For this review, take the finished solid that the model builds, in its own axes (mm). Face numbers are marked on the shaded views. A direction names the side the tool comes from. Round coordinates to 2 decimals unless told otherwise and drop trailing zeros. Loops run counter-clockwise (first coordinate to the right, second up) from the corner with the lowest first, then second, coordinate; pieces in that order, holes last. Notation, with made-up numbers: (4, -5) -> (49, -5) arc R27 cw to (49, 32) -> close; hole circle Ø1 at (-15.75, 45.5). An arc over 180 degrees is marked (long way). Write each question's results on one line, items separated by ' | '.
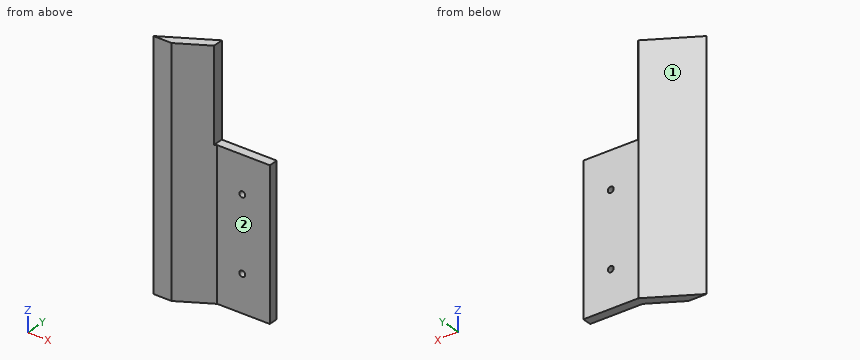
Autodesk Inventor part; units mm, degrees
ref_plane "YZ Plane" through (0, 0, 0) normal (1, 0, 0) x (0, 1, 0)
ref_plane "XZ Plane" through (0, 0, 0) normal (0, 1, 0) x (-1, 0, 0)
ref_plane "XY Plane" through (0, 0, 0) normal (0, 0, 1) x (1, 0, 0)
sketch "スケッチ1" plane through (0, 0, 0) normal (0, 0, 1) x (1, 0, 0)
  line L0 (0, 0) -> (25.9808, 15)
  line L1 (25.9808, 15) -> (55.9808, 15)
  line L2 (55.9808, 15) -> (55.9808, 10)
  line L3 (55.9808, 10) -> (27.3205, 10)
  line L4 (27.3205, 10) -> (10, 0)
  line L5 (10, 0) -> (0, 0)
  dimension "d0" = 15
  dimension "d1" = 5
  dimension "d2" = 5
  dimension "d3" = 30
  dimension "d21" = 30
extrude "押し出し1" add sketch "スケッチ1" along normal blind 130
sketch "スケッチ2" plane through (25.9808, 15, 0) normal (0, 1, 0) x (1, 0, 0)
  line L0 (0.0508, -80) -> (34.0508, -80)
  line L1 (34.0508, -80) -> (34.0508, -130.8394)
  line L2 (34.0508, -130.8394) -> (0.0508, -130.8394)
  line L3 (0.0508, -130.8394) -> (0.0508, -80)
  line L4 (30, 0) -> (0, 0)
  line L5 (30, -130) -> (0, -130)
  point P0 (-25.9808, 0)
  point P1 (15, 0)
  point P2 (17.0508, -130.8394)
  point P3 (15, -130)
  dimension "d7" = 80
  dimension "d22" = 34
extrude "押し出し2" cut sketch "スケッチ2" against normal blind 300
sketch "スケッチ3" plane through (25.9808, 15, 0) normal (0, 1, 0) x (1, 0, 0)
  line L0 (30, 0) -> (30, -130)
  line L1 (30, 0) -> (0, 0)
  line L2 (30, -130) -> (0, -130)
  point P0 (-25.9808, 0)
  point P1 (15, -20)
  point P2 (30, -80)
  point P3 (15, -60)
  point P4 (15, -130)
  dimension "d12" = 15
  dimension "d13" = 20
  dimension "d23" = 40
hole "穴1" at (40.9808, 15, 20) at (40.9808, 15, 60) direction (0, -1, 0) diameter 3.2 depth 10 tip angle 118
properties part number "バンパー1"
1. Tool access review of the marked faces 1 and 2: name each direction out of +Z, -Z, +X, -X, +Y, -Y from which nothing blocks a thin tool from reaching the whole face with its end or side.
Values found:
face 1: +Z, -Z, -X, +Y | face 2: +Z, -Z, +X, -Y
2. Consider section C-C (y = 13). State the section outline as (x, z) points, plus the area to 3 significant figures.
Values found:
outline: (22.52, 0) -> (55.98, 0) -> (55.98, 80) -> (26.03, 80) -> (26.03, 130) -> (22.52, 130) -> close; hole circle Ø3.2 at (40.98, 20); hole circle Ø3.2 at (40.98, 60) | area: 2,840 mm2
3. Consider section B-B (z = 99.5). State the section outline as (x, y) points.
Values found:
outline: (0, 0) -> (10, 0) -> (26.03, 9.26) -> (26.03, 15) -> (25.98, 15) -> close
4. Consider section A-A (z = 60). State the section outline as (x, y) points, plus the area to 3 significant figures.
Values found:
outline: (0, 0) -> (10, 0) -> (27.32, 10) -> (39.38, 10) -> (39.38, 15) -> (25.98, 15) -> close; (42.58, 10) -> (55.98, 10) -> (55.98, 15) -> (42.58, 15) -> close | area: 256 mm2
5. For pin 1 (10 mm diameter, centred on x = 36.5, z = 63.5, fed in from -Y); pin 2 (1.7 mm diameter, centred on y = 11, z = 106, fed in from +X); pin 3 (8 mm diameter, centred on x = 20, y = 5.5, fed in from +Z); pin 4 (2 mm diameter, centred on y = 5.5, z = 37, fed in from +X), all flat-tipped, find the tip position at first contact; note any pin that passes through.
Values found:
pin 1: stops at y = 10 | pin 2: stops at x = 26.03 | pin 3: stops at z = 130 | pin 4: stops at x = 21.26
6. To check wall thickness, follow probe 1 along Z at (x, y) = (41, 11.5); probe 2 along Z at (x, y) = (31.5, 12); probe 3 along X at (y, z) = (12.6, 60). State the ranges of each line that lie inside material, in increasing order.
Values found:
probe 1: z = 0 to 18.4, 21.6 to 58.4, 61.6 to 80 | probe 2: z = 0 to 80 | probe 3: x = 21.82 to 39.38, 42.58 to 55.98
7. Consider section D-D (x = 34). State the section outline as (y, z) points, plus the area to 3 significant figures.
Values found:
outline: (10, 0) -> (15, 0) -> (15, 80) -> (10, 80) -> close | area: 400 mm2
